from build123d import *

# Parameters (mm, degrees)
SKETCH1_W              = 46
SKETCH1_H              = 38
BOSS_EXTRUDE1_DEPTH    = 15
M10X1_0_TAPPED_HOLE1_D = 9
SKETCH7_R              = 7.95
CUT_EXTRUDE1_DEPTH     = 62.522353661
SKETCH17_W             = 38
SKETCH17_H             = 5
BOSS_EXTRUDE2_DEPTH    = 10
SKETCH18_W             = 38
SKETCH18_H             = 5
BOSS_EXTRUDE3_DEPTH    = 10


with BuildPart() as part:
    # Sketch1 → Boss-Extrude1 (new body)
    with BuildSketch(Plane(origin=(0, 0, 0), x_dir=(1, 0, 0), z_dir=(0, 1, 0))):
        with Locations((23, 19)):
            Rectangle(SKETCH1_W, SKETCH1_H)
    extrude(amount=BOSS_EXTRUDE1_DEPTH)

    # M10x1.0 Tapped Hole1 (through all)
    with Locations(Plane(origin=(0, 15, 0), x_dir=(1, 0, 0), z_dir=(0, 1, 0))):
        with Locations((7.5, 29), (38.5, 29), (38.5, 9), (7.5, 9)):
            Hole(M10X1_0_TAPPED_HOLE1_D / 2)

    # Sketch7 → Cut-Extrude1 (cut, through all)
    with BuildSketch(Plane.XY):
        with Locations((23, 15)):
            Circle(SKETCH7_R)
    extrude(amount=-CUT_EXTRUDE1_DEPTH, mode=Mode.SUBTRACT)

    # Sketch17 → Boss-Extrude2 (add)
    with BuildSketch(Plane(origin=(46, 0, 0), x_dir=(0, 0, -1), z_dir=(1, 0, 0))):
        with Locations((19, 2.5)):
            Rectangle(SKETCH17_W, SKETCH17_H)
    extrude(amount=BOSS_EXTRUDE2_DEPTH)

    # Sketch18 → Boss-Extrude3 (add)
    with BuildSketch(Plane.ZY):
        with Locations((-19, 2.5)):
            Rectangle(SKETCH18_W, SKETCH18_H)
    extrude(amount=BOSS_EXTRUDE3_DEPTH)


solid = part.part
CAD build for the part. Positions are in the model's coordinates, mm. A direction names the side the tool comes from. Round coordinates to 2 decimals unless told otherwise and drop trailing zeros. Write each loop counter-clockwise with the first axis right and the second up, starting at its lowest first coordinate (ties: lowest second). Pieces come first, ordered by that corner, then holes.
(1) Slice it at A-A, the plane z = -29. Write the cut outline in (x, y), and give its area (3 significant figures).
(2) Drop flat-ended pins along their axis: P1, Ø3, axis at y = 11.5, z = -30, coming from the -X side; P2, Ø3, axis at y = 11.5, z = -10.5, coming from the +X side; P3, Ø6, axis at x = 19.5, z = -15.5, coming from the +Y side. Give the stop position or say it passes through.
(3) Slice it at C-C, the plane y = 2.5. Write the cut outline in (x, z), and give its area (3 significant figures).
(4) Slice it at B-B, the plane x = 38.5. Write the cut outline in (y, z).
(5) Mould opens along X. For faces 1 (the face through (23, 0, -19)), 2 (the face through (0, 10, -19)), 3 (the face through (46, 10, -19)), 4 (the face through (34.208, 7.395, -10.352)) say: pulls with the +X half, pulls with the -X half, needs draft (parallel to the pull), parting line crosses it, or undercut.
(6) Probe line 1 along Z through (x, y) = (7.5, 4.25); line 2 along X through (y, z) = (7, -29); line 3 along X through (y, z) = (11.75, -27). List the from-to ranges inside material, lowest first.
(7) Slice it at D-D, the plane y = 9.5. Write the cut outline in (x, z), and give its area (3 significant figures).
(8) 3-axis set-ups, long thin cutter, end or side, ignore diameter. For faces 5 (the face through (-5, 5, -19)), 6 (the face through (51, 5, -19)), 7 (the face through (56, 3, -19)): which of +Z, -Z, +X, -X, +Y, -Y reach the whole face in a straight line?
From the geometry:
1. outline: (-10, 0) - (3, 0) - (3, 15) - (0, 15) - (0, 5) - (-10, 5) - close; (12, 0) - (34, 0) - (34, 15) - (30.95, 15) arc R7.95 cw to (15.05, 15) - (12, 15) - close; (43, 0) - (56, 0) - (56, 5) - (46, 5) - (46, 15) - (43, 15) - close
1. area: 421 mm2
2. P1: stops at x = 0
2. P2: stops at x = 46
2. P3: stops at y = 10.42
3. outline: (-10, -38) - (56, -38) - (56, 0) - (-10, 0) - close; hole circle Ø9 at (7.5, -29); hole circle Ø9 at (7.5, -9); hole circle Ø9 at (38.5, -29); hole circle Ø9 at (38.5, -9)
3. area: 2,250 mm2
4. outline: (0, -38) - (15, -38) - (15, -33.5) - (0, -33.5) - close; (0, -24.5) - (15, -24.5) - (15, -13.5) - (0, -13.5) - close; (0, -4.5) - (15, -4.5) - (15, 0) - (0, 0) - close
5. face 1: needs draft
5. face 2: pulls with the -X half
5. face 3: pulls with the +X half
5. face 4: undercut
6. line 1: z = -38 to -33.5, -24.5 to -13.5, -4.5 to 0
6. line 2: x = 0 to 3, 12 to 34, 43 to 46
6. line 3: x = 0 to 3.47, 11.53 to 15.74, 30.26 to 34.47, 42.53 to 46
7. outline: (0, -38) - (17.26, -38) - (17.26, 0) - (0, 0) - close; (28.74, -38) - (46, -38) - (46, 0) - (28.74, 0) - close; hole circle Ø9 at (7.5, -29); hole circle Ø9 at (7.5, -9); hole circle Ø9 at (38.5, -29); hole circle Ø9 at (38.5, -9)
7. area: 1,060 mm2
8. face 5: +Z, -Z, -X, +Y
8. face 6: +Z, -Z, +X, +Y
8. face 7: +Z, -Z, +X, +Y, -Y
